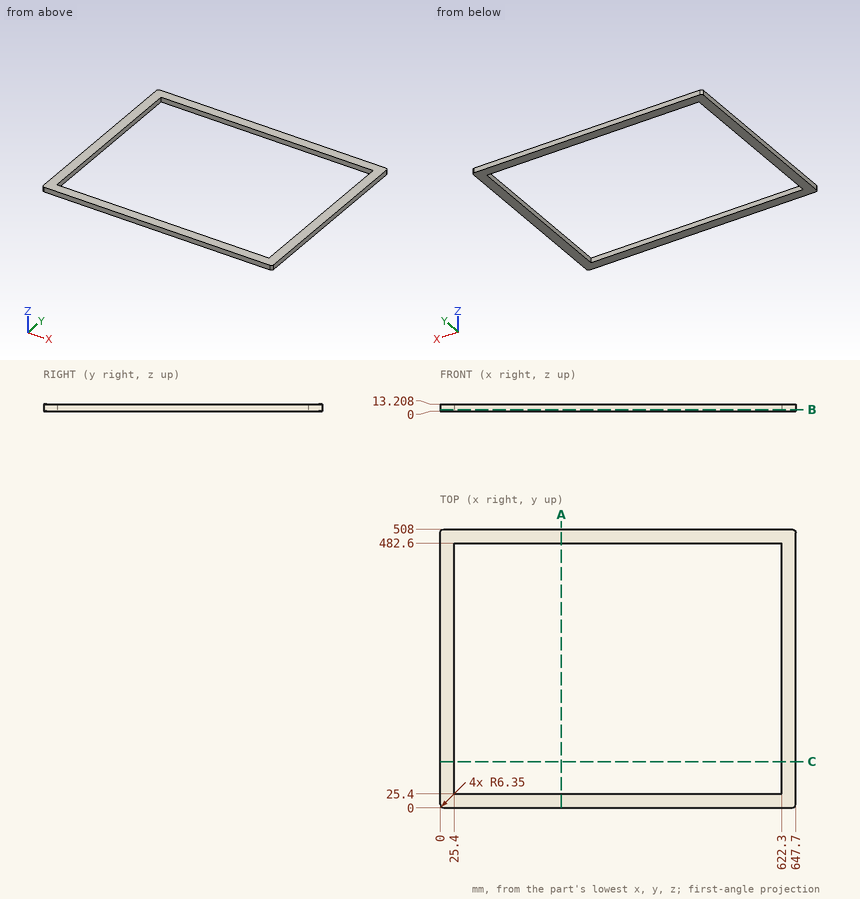
Answer from the drawing. Dimensions are ordinates in mm from the lowest x, y and z of the part. Give positions to 0.01 mm unless a question says otherwise; leave off trailing zeros. Write each loop counter-clockwise with the first axis right and the second up, starting at its lowest first coordinate (ties: lowest second). Pieces come first, ordered by that corner, then holes.
1) Find the intervals of material crossed by L1, parallel to X at y = 42.5, z = 4.5; L2, parallel to Y at x = 335.5, z = 12.5, in increasing order.
2) Section B-B (z = 3) is taken. Write down the section's boundary in (x, y), and give its area (3 significant figures).
3) Section A-A (x = 221) is taken. Write down the section's boundary in (y, z), and give its area (3 significant figures).
4) Section C-C (y = 84.5) is taken. Write down the section's boundary in (x, z).
Response:
1. L1: x = 0 to 25.4, 622.3 to 647.7
1. L2: y = 0 to 25.4, 482.6 to 508
2. outline: (0, 6.35) arc R6.35 ccw to (6.35, 0) - (641.35, 0) arc R6.35 ccw to (647.7, 6.35) - (647.7, 501.65) arc R6.35 ccw to (641.35, 508) - (6.35, 508) arc R6.35 ccw to (0, 501.65) - close; hole (25.4, 25.4) - (622.3, 25.4) - (622.3, 482.6) - (25.4, 482.6) - close
2. area: 56,100 mm2
3. outline: (0, 0) - (25.4, 0) - (25.4, 13.21) - (0, 13.21) - close; (482.6, 0) - (508, 0) - (508, 13.21) - (482.6, 13.21) - close
3. area: 671 mm2
4. outline: (0, 0) - (25.4, 0) - (25.4, 13.21) - (0, 13.21) - close; (622.3, 0) - (647.7, 0) - (647.7, 13.21) - (622.3, 13.21) - close
